```python
from build123d import *

# Parameters (mm, degrees)
CROQUIS1_R              = 1.143
SALIENTE_EXTRUIR8_DEPTH = 3.175


with BuildPart() as part:
    # Croquis1 → Saliente-Extruir8 (new body)
    with BuildSketch(Plane(origin=(0, 0, 0), x_dir=(1, 0, 0), z_dir=(0, 1, 0))):
        with BuildLine():
            ThreePointArc((-16.851199999, 4.270284963), (-19.645199999, 1.476284963), (-16.851199999, -1.317715037))
            add(Edge.make_bspline(
                [(-16.851199999, -1.317715037), (-15.450840408, -1.268925893), (-14.877323423, -1.566939978), (-12.975113768, -2.944503837)],
                knots=[0, 0, 0, 0, 1, 1, 1, 1], degree=3))
            ThreePointArc((-12.975113768, -2.944503837), (-10.120199999, -3.786215037), (-7.265286229, -2.944503837))
            add(Edge.make_bspline(
                [(-7.265286229, -2.944503837), (-5.363076574, -1.566939978), (-4.789559589, -1.268925893), (-3.389199999, -1.317715037)],
                knots=[0.921934519, 0.921934519, 0.921934519, 0.921934519, 1.921934519, 1.921934519, 1.921934519, 1.921934519], degree=3))
            ThreePointArc((-3.389199999, -1.317715037), (-0.595199999, 1.476284963), (-3.389199999, 4.270284963))
            add(Edge.make_bspline(
                [(-3.389199999, 4.270284963), (-4.789559589, 4.221495819), (-5.363076574, 4.519509904), (-7.265286229, 5.897073763)],
                knots=[0, 0, 0, 0, 1, 1, 1, 1], degree=3))
            ThreePointArc((-7.265286229, 5.897073763), (-10.120199999, 6.738784963), (-12.975113768, 5.897073763))
            add(Edge.make_bspline(
                [(-12.975113768, 5.897073763), (-14.877323423, 4.519509904), (-15.450840408, 4.221495819), (-16.851199999, 4.270284963)],
                knots=[0.921934519, 0.921934519, 0.921934519, 0.921934519, 1.921934519, 1.921934519, 1.921934519, 1.921934519], degree=3))
        make_face()
        with Locations((-16.851199999, 1.476284963)):
            Circle(CROQUIS1_R, mode=Mode.SUBTRACT)
        with Locations((-3.389199999, 1.476284963)):
            Circle(CROQUIS1_R, mode=Mode.SUBTRACT)
    extrude(amount=SALIENTE_EXTRUIR8_DEPTH)


solid = part.part
```
The listing builds one solid part. Answer for the finished solid, in the listing's coordinates (mm). Coordinates: 2 decimals unless noted, no trailing zeros. Write each loop counter-clockwise with the first axis right and the second up, starting at its lowest first coordinate (ties: lowest second). Pieces come first, ordered by that corner, then holes. Notation, with made-up numbers: M 88.25,86.25 L 138.25,86.25 A18 ccw 138.25,106.25 Z; hole C 56.25,59 d4. An arc over 180 degrees is marked long. Use a Markdown table: item, result. Add a question column.
1. For a pull along X with two mould halves and no side action, classify faces 1 (the cylindrical face through (-19.645, 1.565, -1.538)), 2 (the cylindrical face through (-0.596, 1.565, -1.415)), 3 (the cylindrical face through (-17.993, 1.565, -1.527)) as +X half, -X half, draft (parallel to the pull), parting line (faces both ways), or undercut.
2. Straight lines are drawn through the part: line 1 along X through (y, z) = (2.75, -1.5); line 2 along X through (y, z) = (1.7, -2); line 3 along X through (y, z) = (3, -3.25). For each, find the intervals that lie inside material, in ascending order. Write a range as [from, to].
3. Section C-C (x = -8.75) is taken. Give the vertices of the cut face in (y, z) (3 decimals).
4. Section B-B (y = 1.95) is taken. Count the separate pieces of the cut face and the enclosed holes in it, plus the area to 3 significant figures.
5. Given P1, Ø4, axis at x = -5, z = -1.5, coming from the -Y side; P2, Ø1.4, axis at x = -16.85, z = -1.48, coming from the +Y side, each flat-ended and moving along its own axis, determine where each tip first touches the part or whether it passes through.
6. Section A-A (z = -0.75) is taken. Give the vertices of the cut face in (x, y) (3 decimals), plus the area to 3 significant figures.
Data:
| question | item | result |
|---|---|---|
| 1 | face 1 | -X half |
| 1 | face 2 | +X half |
| 1 | face 3 | undercut |
| 2 | line 1 | x = [-19.65, -17.99], [-15.71, -4.53], [-2.25, -0.6] |
| 2 | line 2 | x = [-19.6, -17.87], [-15.84, -4.41], [-2.37, -0.64] |
| 2 | line 3 | x = [-19.01, -1.23] |
| 3 | outline | M 0,-6.557 L 3.175,-6.557 L 3.175,3.605 L 0,3.605 Z |
| 4 | separate pieces | 1 |
| 4 | enclosed holes | 2 |
| 4 | area | 125 mm2 |
| 5 | P1 | stops at y = 0 |
| 5 | P2 | passes through |
| 6 | outline | M -19.549,0 L -17.734,0 L -17.734,3.175 L -19.549,3.175 Z; M -15.969,0 L -4.272,0 L -4.272,3.175 L -15.969,3.175 Z; M -2.507,0 L -0.691,0 L -0.691,3.175 L -2.507,3.175 Z |
| 6 | area | 48.7 mm2 |
